Read the model definition and answer for the solid it produces. Units are mm, in the model's axes. A direction names the side the tool comes from. Coordinates: 2 decimals unless noted, no trailing zeros. Loops run counter-clockwise (first coordinate to the right, second up) from the corner with the lowest first, then second, coordinate; pieces in that order, holes last. Notation, with made-up numbers: M 17.25,81 L 25.25,81 A14 ccw 25.25,88 Z; hole C 43.25,66.25 d8. An arc over 180 degrees is marked long. Use one line per item in the form item = value. Start each with the question number.
1. For a pull along X with two mould halves and no side action, classify faces 3 (the cylindrical face through (-53.57, 41.07, 3.7)), 4 (the flat face through (59.824, 11.664, 4.458)) as released by +X, released by -X, zero draft, split by the parting line, or undercut.
2. Find the intervals of material crossed by probe 1 along X at (y, z) = (0.5, 1.75); probe 2 along Y at (x, z) = (0, 5.7); probe 3 along Y at (x, z) = (37, 3), in increasing order. Write a range as [from, to].
3. Flat-ended cylindrical pins translate along their axes: pin 1 (1.5 mm diameter, centred on x = -46, z = 3, fed in from +Y); pin 2 (4 mm diameter, centred on x = -15.5, z = 3.5, fed in from -Y); pin 3 (2 mm diameter, centred on x = -28.5, z = 2, fed in from +Y). Find the tip coordinate at first contact, or state that the pin passes through.
4. The part is cut by section C-C (z = 3.25). Give the number of separate pieces and of enclosed holes in the cut face, plus the area to 3 significant figures.
5. A tool of negligible diameter and unlimited length cuts with its end or side. For faces 1 (the cylindrical face through (-43.25, 33.16, 3.7)), 2 (the flat face through (0, 60, 1.5)), from which of +Z, -Z, +X, -X, +Y, -Y can it reach the whole face along a straight path? Write none if from no direction.
6. The part is cut by section B-B (y = 0). Give the vertices of the cut face in (x, z).
7. The part is cut by section D-D (y = 59.75). Give the vertices of the cut face in (x, z), plus the area to 3 significant figures.
8. The part is cut by section A-A (x = 0). Give the vertices of the cut face in (y, z), plus the area to 3 significant figures.
Autodesk Fusion 360 part; units mm, degrees
sketch "Sketch1" plane through (0, 0, 0) normal (0, 0, 1) x (1, 0, 0)
  circle A0 centre (0, 0) radius 54.5
  circle A1 centre (0, 0) radius 67.5
  line L0 (0, 0) -> (67.5, 0) construction
  line L1 (0, 0) -> (67.5, 0) construction
  line L2 (0, 56.25) -> (0, 63.25) construction
  circle A2 centre (0, 59.75) radius 3
  line L3 (-7.1543, 57.0532) -> (-8.2283, 63.973)
  line L4 (7.0818, 57.0622) -> (7.7138, 64.0371)
  line L5 (-56.4716, 10.8263) -> (-63.3846, 11.9432)
  circle A3 centre (-56.8256, 18.4638) radius 3
  line L6 (-52.081, 24.3683) -> (-58.5192, 27.1248)
  line L7 (-27.7471, -50.3622) -> (-30.9456, -56.5917)
  circle A4 centre (-35.1202, -48.3388) radius 3
  line L8 (-39.2696, -42.0018) -> (-43.8806, -47.273)
  line L9 (39.323, -41.9518) -> (44.2592, -46.9188)
  circle A5 centre (35.1202, -48.3388) radius 3
  line L10 (27.8111, -50.3269) -> (31.3995, -56.3411)
  line L11 (52.05, 24.4345) -> (58.2993, 27.5943)
  circle A6 centre (56.8256, 18.4638) radius 3
  line L12 (56.4578, 10.8981) -> (63.2866, 12.4523)
  arc A7 (52.05, 24.4345) -> (7.0818, 57.0622) centre (0, 0) ccw
  arc A8 (58.2993, 27.5943) -> (7.7138, 64.0371) centre (0, 0) ccw
  arc A9 (-7.1543, 57.0532) -> (-52.081, 24.3683) centre (0, 0) ccw
  arc A10 (-8.2283, 63.973) -> (-58.5192, 27.1248) centre (0, 0) ccw
  arc A11 (-56.4716, 10.8263) -> (-39.2696, -42.0018) centre (0, 0) ccw
  arc A12 (-63.3846, 11.9432) -> (-43.8806, -47.273) centre (0, 0) ccw
  arc A13 (-27.7471, -50.3622) -> (27.8111, -50.3269) centre (0, 0) ccw
  arc A14 (39.323, -41.9518) -> (56.4578, 10.8981) centre (0, 0) ccw
  arc A15 (-30.9456, -56.5917) -> (31.3995, -56.3411) centre (0, 0) ccw
  arc A16 (44.2592, -46.9188) -> (63.2866, 12.4523) centre (0, 0) ccw
  line L13 (0, 0) -> (0, 67.5) construction
  dimension "d1" = 109
  dimension "d2" = 135
  dimension "d3" = 115
  dimension "d4" = 129
  dimension "d7" = 6
  dimension "d8" = 7
  dimension "d10" = 360
  dimension "d11" = 59.75
  dimension "d12" = 14
  dimension "d14" = 7.2954
  dimension "d15" = 14.8681
extrude "Extrude1" add sketch "Sketch1" along normal blind 1.5 contours A2 | L3 L6 A9 A10 | L4 L11 A7 A8 | L5 L8 A11 A12 | A3 | L7 L10 A13 A15 | A4 | L9 L12 A14 A16 | A5 | A6 makes body 1 at (34.6202, -46.3461, 0) makes body 2 at (61.3877, 8.8614, 0) makes body 3 at (-54.8723, 28.9138, 0) makes body 4 at (-44.4551, -43.2519, 0) makes body 5 at (59.8219, 18.3142, 1) makes body 6 at (-53.8294, 18.3142, 1) makes body 7 at (27.3976, -55.6449, 0) makes body 8 at (10.5421, 61.1215, 0) makes body 9 at (-34.2393, -47.0468, 0) makes body 10 at (2.9963, 59.6005, 1)
extrude "Extrude2" add sketch "Sketch1" along normal blind 7.5 bodies 1 2 3 4 5 6 7 8 9 10
Computed values:
q1.face_3 = split by the parting line
q1.face_4 = undercut
q2.probe_1 = [-67.5, -64.5], [-57.5, -54.5], [54.5, 57.5], [64.5, 67.5]
q2.probe_2 = [-67.5, -64.5], [-57.5, -54.5], [54.5, 56.75], [62.75, 67.5]
q2.probe_3 = [-56.46, -50.68], [-46, -40.02], [40.02, 44.01], [52.83, 56.46]
q3.pin_1 = 50.09
q3.pin_2 = -66.14
q3.pin_3 = 61.64
q4.separate_pieces = 1
q4.enclosed_holes = 11
q4.area = 2,690 mm²
q5.face_1 = +Z, -Z
q5.face_2 = +Z
q6.outline = M -67.5,0 L -54.5,0 L -54.5,7.5 L -57.5,7.5 L -57.5,1.5 L -64.5,1.5 L -64.5,7.5 L -67.5,7.5 Z; M 54.5,0 L 67.5,0 L 67.5,7.5 L 64.5,7.5 L 64.5,1.5 L 57.5,1.5 L 57.5,7.5 L 54.5,7.5 Z
q7.outline = M -31.4,0 L 31.4,0 L 31.4,7.5 L 24.29,7.5 L 24.29,1.5 L 7.33,1.5 L 7.33,7.5 L 3,7.5 L 3,1.5 L -3,1.5 L -3,7.5 L -7.57,7.5 L -7.57,1.5 L -24.29,1.5 L -24.29,7.5 L -31.4,7.5 Z
q7.area = 233 mm²
q8.outline = M -67.5,0 L -54.5,0 L -54.5,7.5 L -57.5,7.5 L -57.5,1.5 L -64.5,1.5 L -64.5,7.5 L -67.5,7.5 Z; M 54.5,0 L 67.5,0 L 67.5,7.5 L 62.75,7.5 L 62.75,1.5 L 56.75,1.5 L 56.75,7.5 L 54.5,7.5 Z
q8.area = 117 mm²
